Work out the finished part from the listing and answer in its coordinate system (mm). Coordinates: 2 decimals unless noted, no trailing zeros. Loops run counter-clockwise (first coordinate to the right, second up) from the corner with the lowest first, then second, coordinate; pieces in that order, holes last.
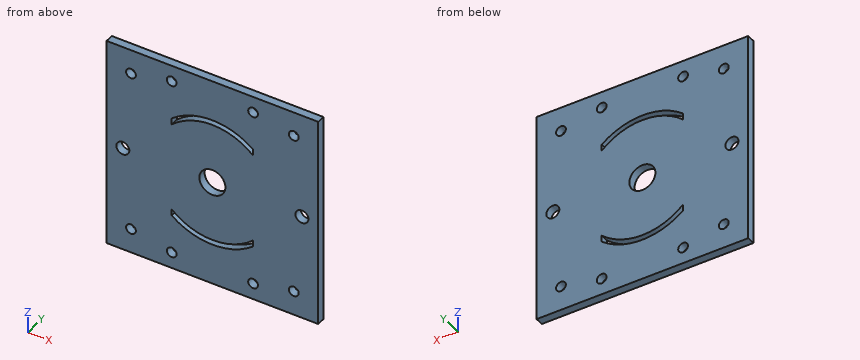
```python
from build123d import *

# Parameters (mm, degrees)
SKETCH1_W           = 130
SKETCH1_H           = 130
SKETCH1_R           = 3
BOSS_EXTRUDE1_DEPTH = 5
SKETCH2_R           = 8
CUT_EXTRUDE1_DEPTH  = 5
SKETCH3_R           = 4
CUT_EXTRUDE2_DEPTH  = 5
SKETCH4_R           = 3
CUT_EXTRUDE3_DEPTH  = 10
CUT_EXTRUDE4_DEPTH  = 10


with BuildPart() as part:
    # Sketch1 → Boss-Extrude1 (new body)
    with BuildSketch(Plane(origin=(0, 0, 0), x_dir=(1, 0, 0), z_dir=(0, 1, 0))):
        Rectangle(SKETCH1_W, SKETCH1_H)
        with Locations(Location((-50, 50, 0), (0, 0, 270))):
            Circle(SKETCH1_R, mode=Mode.SUBTRACT)
        with Locations(Location((50, 50, 0), (0, 0, 90))):
            Circle(SKETCH1_R, mode=Mode.SUBTRACT)
        with Locations(Location((50, -50, 0), (0, 0, 270))):
            Circle(SKETCH1_R, mode=Mode.SUBTRACT)
        with Locations(Location((-50, -50, 0), (0, 0, 90))):
            Circle(SKETCH1_R, mode=Mode.SUBTRACT)
    extrude(amount=BOSS_EXTRUDE1_DEPTH)

    # Sketch2 → Cut-Extrude1 (cut)
    with BuildSketch(Plane(origin=(0, 5, 0), x_dir=(1, 0, 0), z_dir=(0, 1, 0))):
        with Locations(Location((0, 0, 0), (0, 0, 270))):
            Circle(SKETCH2_R)
    extrude(amount=-CUT_EXTRUDE1_DEPTH, mode=Mode.SUBTRACT)

    # Sketch3 → Cut-Extrude2 (cut)
    with BuildSketch(Plane(origin=(0, 5, 0), x_dir=(1, 0, 0), z_dir=(0, 1, 0))):
        with Locations(Location((-55, 0, 0), (0, 0, 270))):
            Circle(SKETCH3_R)
        with Locations(Location((55, 0, 0), (0, 0, 270))):
            Circle(SKETCH3_R)
    extrude(amount=-CUT_EXTRUDE2_DEPTH, mode=Mode.SUBTRACT)

    # Sketch4 → Cut-Extrude3 (cut)
    with BuildSketch(Plane(origin=(0, 5, 0), x_dir=(1, 0, 0), z_dir=(0, 1, 0))):
        with Locations(Location((-25, 55, 0), (0, 0, 270))):
            Circle(SKETCH4_R)
        with Locations(Location((25, 55, 0), (0, 0, 270))):
            Circle(SKETCH4_R)
        with Locations(Location((-25, -55, 0), (0, 0, 270))):
            Circle(SKETCH4_R)
        with Locations(Location((25, -55, 0), (0, 0, 270))):
            Circle(SKETCH4_R)
    extrude(amount=-CUT_EXTRUDE3_DEPTH, mode=Mode.SUBTRACT)

    # Sketch5 → Cut-Extrude4 (cut)
    with BuildSketch(Plane(origin=(0, 5, 0), x_dir=(1, 0, 0), z_dir=(0, 1, 0))):
        with BuildLine():
            Line((25, 31.224989992), (25, 27.276363394))
            ThreePointArc((25, 27.276363394), (0, 37), (-25, 27.276363394))
            Line((-25, 27.276363394), (-25, 31.224989992))
            ThreePointArc((-25, 31.224989992), (0, 40), (25, 31.224989992))
        make_face()
        with BuildLine():
            Line((25, -27.276363394), (25, -31.224989992))
            ThreePointArc((25, -31.224989992), (0, -40), (-25, -31.224989992))
            Line((-25, -31.224989992), (-25, -27.276363394))
            ThreePointArc((-25, -27.276363394), (0, -37), (25, -27.276363394))
        make_face()
    extrude(amount=-CUT_EXTRUDE4_DEPTH, mode=Mode.SUBTRACT)


solid = part.part
```
1. A cutting plane is placed at C-C, the plane z = -6.5. Give the vertices of the cut face in (x, y), then the cut area to 3 significant figures.
2. A cutting plane is placed at B-B, the plane y = 4.2. Count the separate pieces of the cut face and the enclosed holes in it, then the cut area to 3 significant figures.
3. This flat-tipped pin is pushed along its axis until it touches: P1, Ø3.5, axis at x = -25, z = -55, coming from the -Y side. Where does it stop, or does it pass through?
4. A cutting plane is placed at D-D, the plane z = -48.5. Give the vertices of the cut face in (x, y).
5. Straight lines are drawn through the part: probe 1 along X at (y, z) = (2, 55); probe 2 along X at (y, z) = (2.7, 50); probe 3 along X at (y, z) = (3.8, 0). For each, find the intervals that lie inside material, in ascending order.
6. A cutting plane is placed at A-A, the plane z = 50. Give the vertices of the cut face in (x, y), then the cut area to 3 significant figures.
Answers below:
1. outline: (-65, 0) - (-4.66, 0) - (-4.66, 5) - (-65, 5) - close; (4.66, 0) - (65, 0) - (65, 5) - (4.66, 5) - close
1. area: 603 mm2
2. separate pieces: 1
2. enclosed holes: 13
2. area: 16,000 mm2
3. P1: passes through
4. outline: (-65, 0) - (-52.6, 0) - (-52.6, 5) - (-65, 5) - close; (-47.4, 0) - (47.4, 0) - (47.4, 5) - (-47.4, 5) - close; (52.6, 0) - (65, 0) - (65, 5) - (52.6, 5) - close
5. probe 1: x = -65 to -28, -22 to 22, 28 to 65
5. probe 2: x = -65 to -53, -47 to 47, 53 to 65
5. probe 3: x = -65 to -59, -51 to -8, 8 to 51, 59 to 65
6. outline: (-65, 0) - (-53, 0) - (-53, 5) - (-65, 5) - close; (-47, 0) - (47, 0) - (47, 5) - (-47, 5) - close; (53, 0) - (65, 0) - (65, 5) - (53, 5) - close
6. area: 590 mm2
